Autodesk Inventor part; units mm, degrees
ref_plane "Plano de trabajo1" through (60.2171, -17.8462, 0) normal (-1, 0, 0) x (0, 0, 1)
ref_plane "YZ Plane" through (0, 0, 0) normal (1, 0, 0) x (0, 1, 0)
ref_plane "XZ Plane" through (0, 0, 0) normal (0, 1, 0) x (-1, 0, 0)
sketch "Boceto1" plane through (0, 0, 0) normal (0, 0, 1) x (1, 0, 0)
  line L0 (42.7171, -0.3462) -> (13.2171, -0.3462)
  circle A0 centre (37.9098, -17.5) radius 13.97
  line L1 (13.2171, -0.3462) -> (13.2171, -35.3462)
  line L2 (13.2171, -0.3462) -> (13.2171, -35.3462)
  line L3 (13.2171, -35.3462) -> (42.7171, -35.3462)
  arc A1 (42.7171, -35.3462) -> (42.7171, -0.3462) centre (42.7171, -17.8462) ccw
  circle A2 centre (37.9098, -17.5) radius 6
  circle A3 centre (37.9098, -17.5) radius 12.5
  circle A4 centre (29.4098, -17.5) radius 1.5
  circle A5 centre (46.4098, -17.5) radius 1.5
  line L4 (22.4098, -0.3462) -> (22.4098, -35.3462)
  line L5 (22.4098, -0.3462) -> (13.2171, -0.3462)
  circle A6 centre (17.8135, -7.8462) radius 2
  circle A7 centre (17.8135, -27.8462) radius 2
  circle A8 centre (17.8135, -7.8462) radius 3.5
  circle A9 centre (17.8135, -27.8462) radius 3.5
  point P0 (0, 0)
  point P1 (38.7171, -2.3462)
  point P2 (38.7171, -33.3462)
  dimension "d4" = 2
  dimension "d5" = 27.94
  dimension "d7" = 33
  dimension "d10" = 12
  dimension "d11" = 25
  dimension "d27" = 4
  dimension "d28" = 4
  dimension "d30" = 20
  dimension "d31" = 7.5
  dimension "d32" = 7
  dimension "d33" = 7
extrude "Extrusión1" add sketch "Boceto1" along normal blind 20.2 contours A1 L3 L4 L0
extrude "Extrusión2" add sketch "Boceto1" along normal blind 20.2 contours L4 L3 L1 L0
extrude "Extrusión3" add sketch "Boceto1" along normal blind 9 contours A8 | A9
extrude "Extrusión4" add sketch "Boceto1" along normal blind 13.2 contours A0
extrude "Extrusión5" add sketch "Boceto1" along normal blind 3 contours A3
sketch "Boceto2" plane through (13.2171, -35.3462, 0) normal (-1, 0, 0) x (0, 0, 1)
  point P0 (0, 35.3462)
ref_plane "Plano de trabajo1" through (60.2171, -17.8462, 0) normal (-1, 0, 0) x (0, 0, 1)
sketch "Boceto3" plane through (60.2171, -17.8462, 0) normal (-1, 0, 0) x (0, 0, 1)
  line L0 (20.2, -17.5) -> (20.2, 17.5)
  line L1 (20.2, 0) -> (9.2, 0)
  circle A0 centre (9.2, 0) radius 3.5
  point P0 (0, 17.8462)
  dimension "d44" = 11
  dimension "d45" = 7
hole "Agujero1" at (60.2171, -17.8462, 9.2) direction (-1, 0, 0) diameter 7 end through all
fillet "Empalme1" radius 2 3 edges at (27.9671, -0.3462, 0) (27.9671, -35.3462, 0) (60.2171, -17.8462, 0)
fillet "Empalme2" radius 0.5 1 edges at (31.9098, -17.5, 0)
fillet "Empalme3" radius 0.5 1 edges at (23.9398, -17.5, 20.2)
fillet "Empalme4" radius 0.5 1 edges at (14.3135, -7.8462, 20.2)
fillet "Empalme5" radius 0.5 1 edges at (14.3135, -27.8462, 20.2)
properties part number "Rodamiento grande"
Input: part model. Units: mm. Frame: model coordinates. A direction names the side the tool comes from. Give positions to 0.01 mm unless a question says otherwise; leave off trailing zeros. Loops run counter-clockwise (first coordinate to the right, second up) from the corner with the lowest first, then second, coordinate; pieces in that order, holes last. Notation, with made-up numbers: (-20.5, -31) -> (36.5, -31) arc R33 cw to (36.5, 1) -> close; hole circle Ø3 at (45, -18). An arc over 180 degrees is marked (long way). Answer as a JSON object with one key per item and string values. Group by question number.
Item 1: Pin query (flat end, axial travel): P1, Ø7.5, axis at x = 19, y = -26.5, coming from the +Z side; P2, Ø8.5, axis at x = 31.5, y = -23, coming from the +Z side; P3, Ø1.5, axis at y = -8, z = 17, coming from the +X side; P4, Ø15.5, axis at x = 37.91, y = -17.5, coming from the +Z side. Return the tip coordinate at first contact, or that it passes through.
Item 2: Cut plane B-B, the plane x = 18.5. State how many separate pieces and enclosed holes the cut face has, and give its area (3 significant figures).
Item 3: Cut plane A-A, the plane z = 15.5. Return the cut outline in (x, y), and give its area (3 significant figures).
Item 4: Pull-direction query (X, two-part tool) for faces 3 (the flat face through (13.217, -14, 10)), 4 (the cylindrical face through (44.36, -5.11, 16.4)), 5 (the cylindrical face through (28.174, -34.776, 0.601)), 6 (the flat face through (19.3, -9.4, 9)); classes: released by +X, released by -X, zero draft, split by the parting line, or undercut.
Item 5: Reachability of faces 1 (the flat face through (47, -29, 20.2)), 2 (the flat face through (27, -25, 13.2)) from +Z, -Z, +X, -X, +Y, -Y: full face, straight path, thin tool, end or side. Return the list, or none.
Item 6: Line query: probe 1 along Y at (x, z) = (18, 9.2); probe 2 along X at (y, z) = (-28, 15.5); probe 3 along Y at (x, z) = (18, 7.25). Output: solid intervals per line, ascending.
Checks:
{
 "1": {"P1": "stops at z = 20.2", "P2": "stops at z = 13.2", "P3": "stops at x = 57.67", "P4": "stops at z = 3"},
 "2": {"separate pieces": "3", "enclosed holes": "1", "area": "445 mm²"},
 "3": {"outline": "(13.22, -35.35) -> (42.72, -35.35) arc R17.5 ccw to (42.72, -0.35) -> (13.22, -0.35) -> close; hole circle Ø7 at (17.81, -27.85); hole circle Ø7 at (17.81, -7.85); hole circle Ø27.94 at (37.91, -17.5)", "area": "823 mm²"},
 "4": {"face 3": "released by -X", "face 4": "undercut", "face 5": "zero draft", "face 6": "undercut"},
 "5": {"face 1": "+Z, +X, -X, +Y, -Y", "face 2": "+Z"},
 "6": {"probe 1": "y = -35.35 to -31.34, -24.35 to -21.35, -14.35 to -11.34, -4.35 to -0.35", "probe 2": "x = 13.22 to 14.32, 21.31 to 28.7, 47.12 to 56.97", "probe 3": "y = -35.35 to -29.84, -25.85 to -20.75, -14.94 to -9.84, -5.85 to -0.35"}
}
